Part model, mm, in its own coordinate system. Coordinates: 2 decimals unless noted, no trailing zeros. Order: outer loops, then holes, each group sorted by start corner. A loop starts at its lowest first (then second) coordinate and runs counter-clockwise, first axis right, second up. Notation, with made-up numbers: (47, 18) - (83, 18) arc R10 cw to (83, 37) - close; hole circle Ø5 at (71, -11.75). An arc over 180 degrees is marked (long way). Use a Markdown table: item, result. Add a question column.
1) Saw through at A-A on x = 0. List the corners of the cut face in (y, z).
2) Drop flat-ended pins along their axis: P1, Ø8, axis at x = -62.5, y = -44, coming from the -Z side; P2, Ø2, axis at y = 54, z = 2.5, coming from the +X side; P3, Ø1, axis at y = 3.5, z = 4.5, coming from the -X side; P4, Ø5, axis at x = -3, y = 66, coming from the -Z side. Give the stop position or say it passes through.
3) Saw through at B-B on y = 0. List the corners of the cut face in (x, z), then the cut area to 3 significant figures.
4) Wall check: L1, parallel to Y at x = 0, z = 4.05; L2, parallel to X at y = 24, z = 1.25; L3, parallel to Y at x = -0.5, z = 1.5. Give the ranges that are in metal, low to high. Write a range as [from, to].
5) Saw through at C-C on z = 4. Count the separate pieces of the cut face and the enclosed holes in it, then the cut area to 3 significant figures.
```python
from build123d import *

# Parameters (mm, degrees)
SKETCH1_R                                        = 127
SKETCH1_R_2                                      = 52.07
BOSS_EXTRUDE1_DEPTH                              = 6.35
CBORE_FOR_3_8_SOCKET_HEAD_CAP_SCREW1_D           = 9.9314
CBORE_FOR_3_8_SOCKET_HEAD_CAP_SCREW1_CBORE_D     = 15.875
CBORE_FOR_3_8_SOCKET_HEAD_CAP_SCREW1_CBORE_DEPTH = 1.5494
CIRPATTERN1_COUNT                                = 5
CUT_EXTRUDE1_DEPTH                               = 180.717340566
FILLET1_R                                        = 1


with BuildPart() as part:
    # Sketch1 → Boss-Extrude1 (new body)
    with BuildSketch(Plane.XY):
        Circle(SKETCH1_R)
        Circle(SKETCH1_R_2, mode=Mode.SUBTRACT)
    extrude(amount=BOSS_EXTRUDE1_DEPTH)

    # CBORE for 3/8 Socket Head Cap Screw1 (through all)
    with Locations(Plane(origin=(0, 0, 0), x_dir=(-1, 0, 0), z_dir=(0, 0, -1))):
        with Locations((0, 63.5)):
            cbore_for_3_8_socket_head_cap_screw1 = CounterBoreHole(CBORE_FOR_3_8_SOCKET_HEAD_CAP_SCREW1_D / 2, CBORE_FOR_3_8_SOCKET_HEAD_CAP_SCREW1_CBORE_D / 2, CBORE_FOR_3_8_SOCKET_HEAD_CAP_SCREW1_CBORE_DEPTH)

    # CirPattern1: CBORE for 3/8 Socket Head Cap Screw1 ×5 about axis
    cirpattern1_axis = Axis((0, 0, 0), (0, 0, 1))
    for i in range(1, CIRPATTERN1_COUNT):
        add(cbore_for_3_8_socket_head_cap_screw1.rotate(cirpattern1_axis, i * 360 / CIRPATTERN1_COUNT), mode=Mode.SUBTRACT)

    # Sketch5 → Cut-Extrude1 (cut, through all)
    with BuildSketch(Plane(origin=(0, 0, 0), x_dir=(-1, 0, 0), z_dir=(0, 0, -1))):
        with BuildLine():
            ThreePointArc((-41.44563977, 78.647752314), (-52.234106188, 71.936139393), (-61.955600498, 63.755106203))
            ThreePointArc((-61.955600498, 63.755106203), (-67.246233615, 46.459424342), (-55.472312316, 32.729668808))
            ThreePointArc((-55.472312316, 32.729668808), (-49.895894595, 28.887022327), (-46.775498841, 22.876573349))
            ThreePointArc((-46.775498841, 22.876573349), (-49.521512803, 16.090514897), (-51.28868592, 8.986411775))
            ThreePointArc((-51.28868592, 8.986411775), (-57.354131533, 5.956167187), (-64.132133316, 6.131394358))
            ThreePointArc((-64.132133316, 6.131394358), (-81.713776835, 1.96678681), (-87.605864362, -15.11365374))
            ThreePointArc((-87.605864362, -15.11365374), (-84.556560625, -27.448097481), (-79.780042652, -39.22186628))
            ThreePointArc((-79.780042652, -39.22186628), (-64.965767259, -49.598217006), (-48.269652019, -42.64328022))
            ThreePointArc((-48.269652019, -42.64328022), (-42.8918702, -38.527234874), (-36.211338216, -37.416893037))
            ThreePointArc((-36.211338216, -37.416893037), (-30.605978087, -42.125514897), (-24.395661045, -46.001485))
            ThreePointArc((-24.395661045, -46.001485), (-23.388052957, -52.706463648), (-25.649221638, -59.098578238))
            ThreePointArc((-25.649221638, -59.098578238), (-27.121471128, -77.106649381), (-12.69776202, -87.98850402))
            ThreePointArc((-12.69776202, -87.98850402), (-0.02472225, -88.899996562), (12.648822515, -87.995552666))
            ThreePointArc((12.648822515, -87.995552666), (27.095181344, -77.112808233), (25.640026743, -59.084665376))
            ThreePointArc((25.640026743, -59.084665376), (23.38726097, -52.698162972), (24.395661045, -46.001485))
            ThreePointArc((24.395661045, -46.001485), (30.605978087, -42.125514897), (36.211338216, -37.416893037))
            ThreePointArc((36.211338216, -37.416893037), (42.899519875, -38.530553149), (48.280042559, -42.656324396))
            ThreePointArc((48.280042559, -42.656324396), (64.951785852, -49.621316886), (79.758215853, -39.266232363))
            ThreePointArc((79.758215853, -39.266232363), (84.541281434, -27.495121994), (87.597444884, -15.162376126))
            ThreePointArc((87.597444884, -15.162376126), (81.711510261, 1.939880549), (64.116060019, 6.126948804))
            ThreePointArc((64.116060019, 6.126948804), (57.345992383, 5.957979013), (51.28868592, 8.986411775))
            ThreePointArc((51.28868592, 8.986411775), (49.521512803, 16.090514897), (46.775498841, 22.876573349))
            ThreePointArc((46.775498841, 22.876573349), (49.901414341, 28.893272197), (55.487928918, 32.735519927))
            ThreePointArc((55.487928918, 32.735519927), (67.263882415, 46.438988979), (61.991050299, 63.720637809))
            ThreePointArc((61.991050299, 63.720637809), (52.274107628, 71.907076645), (41.48937575, 78.62468887))
            ThreePointArc((41.48937575, 78.62468887), (23.405309269, 78.311720347), (13.985877573, 62.871327984))
            ThreePointArc((13.985877573, 62.871327984), (12.054511442, 56.380396507), (7.302490092, 51.555392913))
            ThreePointArc((7.302490092, 51.555392913), (0, 52.07), (-7.302490092, 51.555392913))
            ThreePointArc((-7.302490092, 51.555392913), (-12.058749726, 56.387577413), (-13.986616522, 62.88798835))
            ThreePointArc((-13.986616522, 62.88798835), (-23.380420305, 78.322190478), (-41.44563977, 78.647752314))
        make_face()
    extrude(amount=-CUT_EXTRUDE1_DEPTH, mode=Mode.SUBTRACT)

    # Fillet1
    fillet1_edges = [part.edges().sort_by_distance(p)[0] for p in [
        (-127, 0, 0),
        (-127, 0, 6.35),
    ]]
    fillet(fillet1_edges, radius=FILLET1_R)


solid = part.part
```
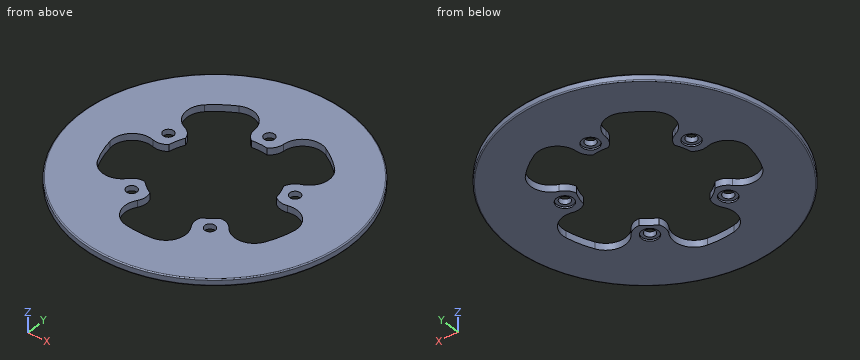
Results are:
| question | item | result |
|---|---|---|
| 1 | outline | (-127, 1) arc R1 ccw to (-126, 0) - (-88.9, 0) - (-88.9, 6.35) - (-126, 6.35) arc R1 ccw to (-127, 5.35) - close; (52.07, 0) - (55.56, 0) - (55.56, 1.55) - (58.53, 1.55) - (58.53, 6.35) - (52.07, 6.35) - close; (68.47, 1.55) - (71.44, 1.55) - (71.44, 0) - (126, 0) arc R1 ccw to (127, 1) - (127, 5.35) arc R1 ccw to (126, 6.35) - (68.47, 6.35) - close |
| 2 | P1 | through |
| 2 | P2 | x = 115.41 |
| 2 | P3 | x = -126.96 |
| 2 | P4 | z = 1.55 |
| 3 | outline | (-127, 1) arc R1 ccw to (-126, 0) - (-83.57, 0) - (-83.57, 6.35) - (-126, 6.35) arc R1 ccw to (-127, 5.35) - close; (83.59, 0) - (126, 0) arc R1 ccw to (127, 1) - (127, 5.35) arc R1 ccw to (126, 6.35) - (83.59, 6.35) - close |
| 3 | area | 551 mm2 |
| 4 | L1 | [-127, -88.9], [52.07, 58.53], [68.47, 127] |
| 4 | L2 | [-124.71, -67.01], [-53.77, -47.09], [47.09, 53.77], [67.01, 124.71] |
| 4 | L3 | [-127, -88.9], [52.07, 55.58], [71.42, 127] |
| 5 | separate pieces | 1 |
| 5 | enclosed holes | 6 |
| 5 | area | 32,100 mm2 |
